```python
from build123d import *

# Parameters (mm, degrees)
F0_W      = 40
F0_H      = 500
F1_DEPTH  = 3
F3_D      = 12
F5_D      = 12
F7_DEPTH  = 6
F8_D      = 12
F10_DEPTH = 6
F12_D     = 6
F13_R     = 5


with BuildPart() as f1:
    # F0 (on Front) → F1 (new body)
    with BuildSketch(Plane.XZ):
        Rectangle(F0_W, F0_H)
    extrude(amount=F1_DEPTH)

    # F3 (through all)
    with Locations(Plane.XZ.offset(3)):
        with Locations((0, -215), (0, 215)):
            Hole(F3_D / 2)

    # F5 (through all)
    with Locations(Plane.XZ.offset(3)):
        with Locations((0, 147)):
            Hole(F5_D / 2)

    # F6 (on face) → F7 (cut)
    with BuildSketch(Plane.XZ.offset(3)):
        with BuildLine():
            ThreePointArc((-3, 153), (0, 150), (3, 153))
            Line((3, 153), (3, 173))
            ThreePointArc((3, 173), (0, 176), (-3, 173))
            Line((-3, 173), (-3, 153))
        make_face()
    extrude(amount=-F7_DEPTH, mode=Mode.SUBTRACT)

    # F8 (through all)
    with Locations(Plane.XZ.offset(3)):
        with Locations((0, -178.25)):
            Hole(F8_D / 2)

    # F9 (on face) → F10 (cut)
    with BuildSketch(Plane.XZ.offset(3)):
        with BuildLine():
            ThreePointArc((-3, -172.25), (0, -175.25), (3, -172.25))
            Line((3, -172.25), (3, -152.25))
            ThreePointArc((3, -152.25), (0, -149.25), (-3, -152.25))
            Line((-3, -152.25), (-3, -172.25))
        make_face()
    extrude(amount=-F10_DEPTH, mode=Mode.SUBTRACT)

    # F12 (through all)
    with Locations(Plane.XZ.offset(3)):
        with Locations((0, 20), (0, -20)):
            Hole(F12_D / 2)

    # F13
    f13_edges = [f1.edges().sort_by_distance(p)[0] for p in [
        (-20, -1.5, -250),
        (20, -1.5, -250),
        (20, -1.5, 250),
        (-20, -1.5, 250),
    ]]
    fillet(f13_edges, radius=F13_R)


solid = f1.part
```
CAD build for the part. Positions are in the model's coordinates, mm. Give positions to 0.01 mm unless a question says otherwise; leave off trailing zeros. Loops run counter-clockwise (first coordinate to the right, second up) from the corner with the lowest first, then second, coordinate; pieces in that order, holes last. Notation, with made-up numbers: (37, 15) - (96, 15) arc R25 ccw to (96, 40) - close; hole circle Ø8 at (66.25, 15). An arc over 180 degrees is marked (long way). Put each result on its own line as item: value.
Q1. Mould opens along Z. For faces 1 (the face through (0.221, -1.479, -184.246)), 2 (the face through (0, -3, 4)), 3 (the face through (1.301, -1.479, -220.857)) say: pulls with the +Z half, pulls with the -Z half, needs draft (parallel to the pull), parting line crosses it, or undercut.
Filled in:
face 1: undercut
face 2: needs draft
face 3: undercut
Q2. Probe line 1 along X through (y, z) = (-1.9, 147); line 2 along X through (y, z) = (-0.9, 159); line 3 along Z through (x, y) = (5, -1.9). List the from-to ranges inside material, lowest first.
Filled in:
line 1: x = -20 to -6, 6 to 20
line 2: x = -20 to -3, 3 to 20
line 3: z = -250 to -218.32, -211.68 to -181.57, -174.93 to 143.68, 150.32 to 211.68, 218.32 to 250
Q3. Slice it at A-A (z = -215). Give the cut face in (x, y).
Filled in:
outline: (-20, -3) - (-6, -3) - (-6, 0) - (-20, 0) - close; (6, -3) - (20, -3) - (20, 0) - (6, 0) - close
Q4. Flat gauge pin, fed straight in: pin 1 (5 mm diameter, centred on x = 0, z = -20, fed in from +Y). Where does the tip first touch, or does it go through?
Filled in:
pin 1: passes through
Q5. Slice it at B-B (y = -1.25). Give the cut face in (x, z), plus the area to 3 significant figures.
Filled in:
outline: (-20, -245) arc R5 ccw to (-15, -250) - (15, -250) arc R5 ccw to (20, -245) - (20, 245) arc R5 ccw to (15, 250) - (-15, 250) arc R5 ccw to (-20, 245) - close; hole circle Ø12 at (0, -215); hole circle Ø12 at (0, 215); hole (-3, -172.25) arc R3 ccw to (-2.9, -173) arc R6 ccw (long way) to (2.9, -173) arc R3 ccw to (3, -172.25) - (3, -152.25) arc R3 ccw to (-3, -152.25) - close; hole circle Ø6 at (0, -20); hole circle Ø6 at (0, 20); hole (-3, 153) arc R3 ccw to (-2.9, 152.25) arc R6 ccw (long way) to (2.9, 152.25) arc R3 ccw to (3, 153) - (3, 173) arc R3 ccw to (-3, 173) - close
area: 19,200 mm²
